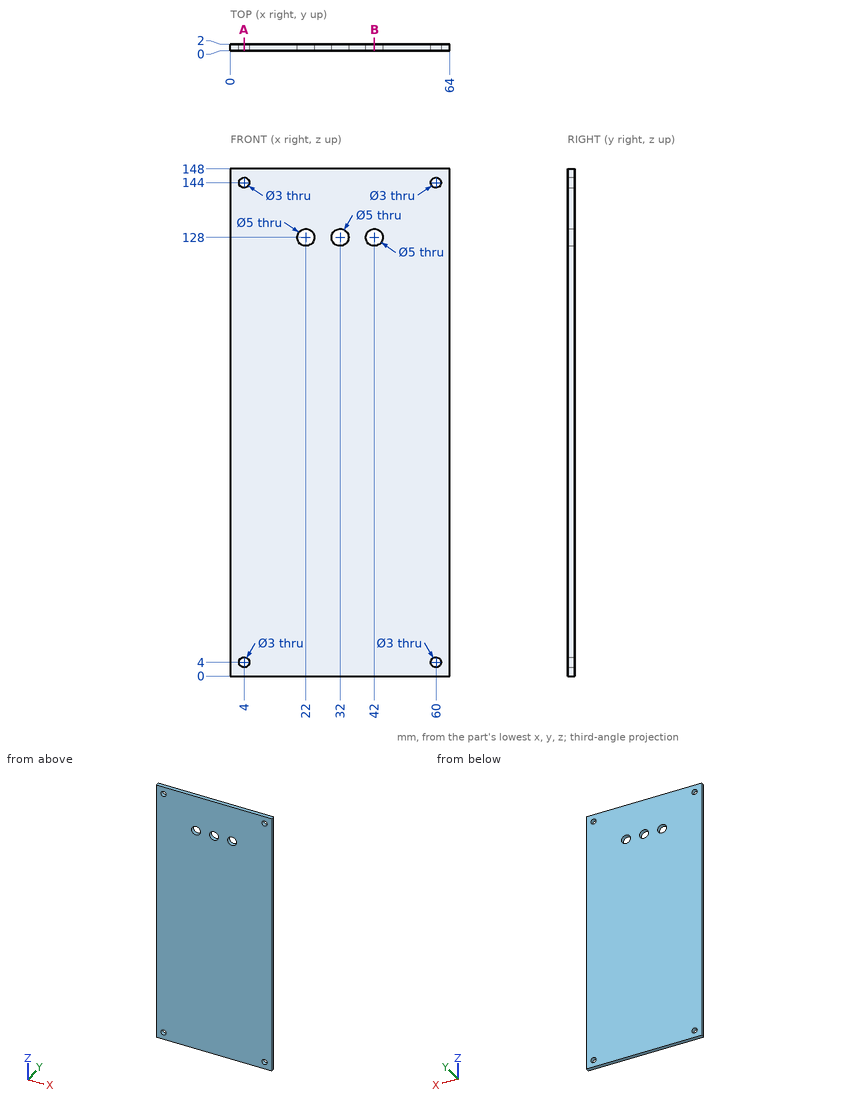
Geometry check sheet. Reference: drawing and pictorial views, mm from the part's lowest x, y, z. Coordinates: 2 decimals unless noted, no trailing zeros. Order: outer loops, then holes, each group sorted by start corner. A loop starts at its lowest first (then second) coordinate and runs counter-clockwise, first axis right, second up. Notation, with made-up numbers: (17, -40) -> (34, -40) arc R34 ccw to (34, -8) -> close; hole circle Ø1 at (65.25, 49.25). An arc over 180 degrees is marked (long way). Write item = value, one per line. Start each with the question number.
1) Go/stop test with a flat-tipped pin: P1, Ø1, axis at x = 41.5, z = 92, coming from the -Y side. Record where the tip stops, or that it passes through.
2) Material ranges on L1, parallel to X at y = 0.85, z = 128; L2, parallel to X at y = 1.5, z = 144; L3, parallel to Z at x = 60, y = 0.8, recorded low to high.
3) Cross-section at A-A (x = 4). Enter the section's corners in (y, z).
4) Cross-section at B-B (x = 42). Enter the section's corners in (y, z), then the cut area to 3 significant figures.
Ans:
q1.P1 = 0
q2.L1 = 0 to 19.5, 24.5 to 29.5, 34.5 to 39.5, 44.5 to 64
q2.L2 = 0 to 2.5, 5.5 to 58.5, 61.5 to 64
q2.L3 = 0 to 2.5, 5.5 to 142.5, 145.5 to 148
q3.outline = (0, 0) -> (2, 0) -> (2, 2.5) -> (0, 2.5) -> close; (0, 5.5) -> (2, 5.5) -> (2, 142.5) -> (0, 142.5) -> close; (0, 145.5) -> (2, 145.5) -> (2, 148) -> (0, 148) -> close
q4.outline = (0, 0) -> (2, 0) -> (2, 125.5) -> (0, 125.5) -> close; (0, 130.5) -> (2, 130.5) -> (2, 148) -> (0, 148) -> close
q4.area = 286 mm²
